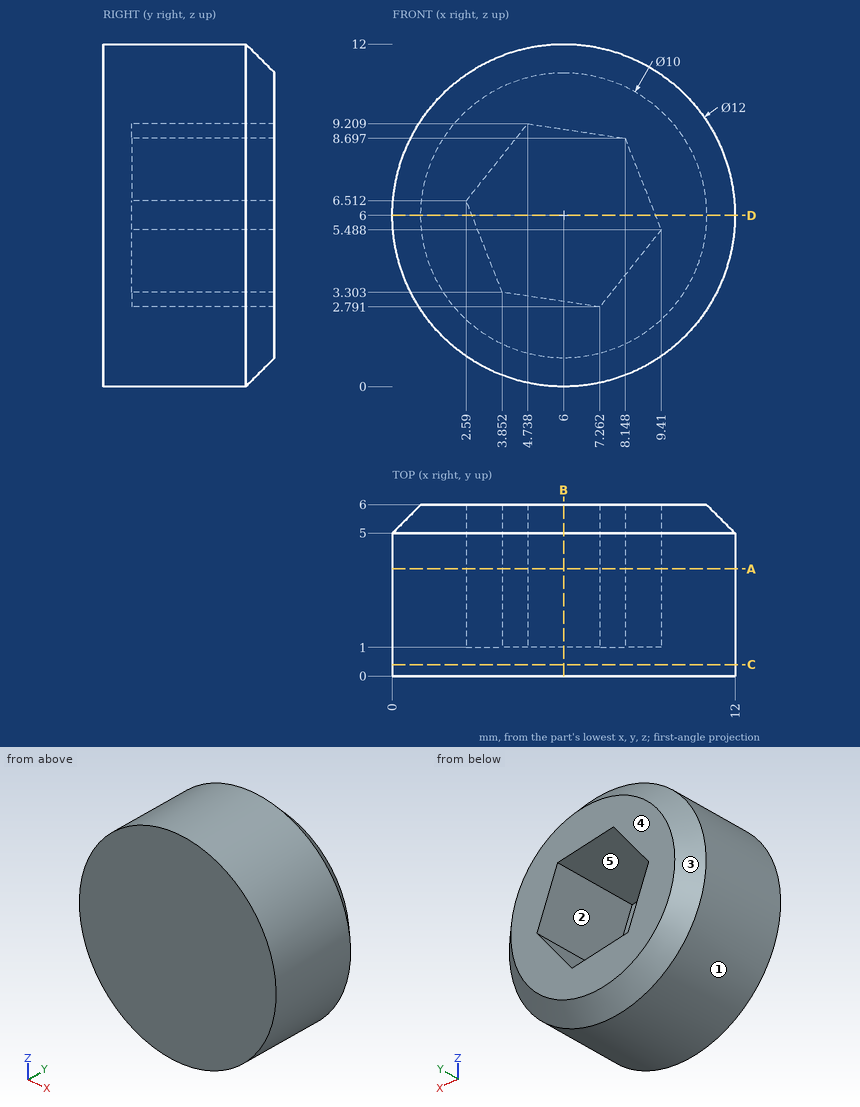
Could you check a few things on this drawing? It's one solid part, dimensions in mm from its lowest x, y, z. A direction names the side the tool comes from. Coordinates: 2 decimals unless noted, no trailing zeros. Loops run counter-clockwise (first coordinate to the right, second up) from the corner with the lowest first, then second, coordinate; pieces in that order, holes last.
1. For the marked faces 1 and 2, which set-ups out of +Z, -Z, +X, -X, +Y, -Y let a thin tool reach every point of the face, with its end or its side?
2. We'd pull the mould along X, two halves only. Please class the marked faces 3, 4 and 5: released by +X, released by -X, zero draft, split by the parting line, or undercut.
3. Imagine slicing it at D-D (z = 6). Please give me the cut outline in (x, y).
4. For P1, Ø3, axis at x = 6, z = 7, coming from the +Y side; P2, Ø1.5, axis at y = 4.5, z = 4.5, coming from the -X side; P3, Ø2, axis at y = 5.5, z = 10, coming from the -X side (1 decimal), each with a flat end and sliding along its axis, tell me the tip position at first contact or that it passes through.
5. I need wall thicknesses on L1, parallel to X at y = 3.25, z = 7 (1 decimal); L2, parallel to X at y = 2.45, z = 3.75 (1 decimal); L3, parallel to Y at x = 8, z = 4.25. Which ranges of each line are inside material? Lowest first, please.
6. Imagine slicing it at B-B (x = 6). Please give me the cut outline in (y, z), and give its area (3 significant figures).
7. Imagine slicing it at A-A (y = 3.75). Please give me the cut outline in (x, z).
8. Imagine slicing it at C-C (y = 0.4). Please give me the cut outline in (x, z), and give its area (3 significant figures).
Computed values:
1. face 1: +Y, -Y
1. face 2: +Y
2. face 3: split by the parting line
2. face 4: zero draft
2. face 5: undercut
3. outline: (0, 0) - (12, 0) - (12, 5) - (11, 6) - (9.21, 6) - (9.21, 1) - (2.79, 1) - (2.79, 6) - (1, 6) - (0, 5) - close
4. P1: stops at y = 1
4. P2: stops at x = 0.05
4. P3: stops at x = 0.9
5. L1: x = 0.1 to 3, 8.8 to 11.9
5. L2: x = 0.4 to 3.7, 8 to 11.6
5. L3: y = 0 to 1
6. outline: (0, 0) - (5, 0) - (6, 1) - (6, 2.98) - (1, 2.98) - (1, 9.02) - (6, 9.02) - (6, 11) - (5, 12) - (0, 12) - close
6. area: 40.8 mm2
7. outline: circle Ø12 at (6, 6); hole (2.59, 6.51) - (3.85, 3.3) - (7.26, 2.79) - (9.41, 5.49) - (8.15, 8.7) - (4.74, 9.21) - close
8. outline: circle Ø12 at (6, 6)
8. area: 113 mm2
